Work out the finished part from the listing and answer in its coordinate system (mm). Coordinates: 2 decimals unless noted, no trailing zeros. Loops run counter-clockwise (first coordinate to the right, second up) from the corner with the lowest first, then second, coordinate; pieces in that order, holes last.
```python
from build123d import *

# Parameters (mm, degrees)
F0_W     = 75
F0_H     = 40
F1_DEPTH = 3
F3_D     = 5.5
F4_D     = 3.3


with BuildPart() as f1:
    # F0 (on Front) → F1 (new body)
    with BuildSketch(Plane.XZ):
        with Locations((37.5, 20)):
            Rectangle(F0_W, F0_H)
    extrude(amount=-F1_DEPTH)

    # F3 (through all)
    with Locations(Plane.XZ):
        with Locations((12.5, 5), (62.5, 5)):
            Hole(F3_D / 2)

    # F4 (through all)
    with Locations(Plane.XZ):
        with Locations((11.75, 36.590098), (31.05, 36.590098), (43.94, 36.590098), (63.24, 36.590098)):
            Hole(F4_D / 2)


solid = f1.part
```
1. Straight lines are drawn through the part: probe 1 along X at (y, z) = (1.05, 36.5); probe 2 along Z at (x, y) = (62, 2.35); probe 3 along Z at (x, y) = (12.5, 1.3). For each, find the intervals that lie inside material, in ascending order.
2. A cutting plane is placed at D-D, the plane y = 1.7. Give the vertices of the cut face in (x, z).
3. A cutting plane is placed at B-B, the plane z = 7. Give the vertices of the cut face in (x, y).
4. Each of these flat-tipped pins is pushed along its axis until it touches: P1, Ø4.5, axis at x = 43.94, z = 36.59, coming from the +Y side; P2, Ø2, axis at x = 63.24, z = 36.59, coming from the -Y side (3 decimals). Where does it stop, or does it pass through?
5. A cutting plane is placed at A-A, the plane x = 43.94. Give the vertices of the cut face in (y, z), then the cut area to 3 significant figures.
6. A cutting plane is placed at C-C, the plane x = 63.24. Give the vertices of the cut face in (y, z), then the cut area to 3 significant figures.
7. Determine the mould class of faces 1 (the flat face through (0, 1, 20)), 2 (the cylindrical face through (32.266, 1.521, 37.705)), 3 (the flat face through (37, 1, 40)) for opening direction X: released by +X, released by -X, zero draft, split by the parting line, or undercut.
Answers below:
1. probe 1: x = 0 to 10.1, 13.4 to 29.4, 32.7 to 42.29, 45.59 to 61.59, 64.89 to 75
1. probe 2: z = 0 to 2.3, 7.7 to 35.5, 37.68 to 40
1. probe 3: z = 0 to 2.25, 7.75 to 35.12, 38.06 to 40
2. outline: (0, 0) - (75, 0) - (75, 40) - (0, 40) - close; hole circle Ø5.5 at (12.5, 5); hole circle Ø3.3 at (11.75, 36.59); hole circle Ø3.3 at (31.05, 36.59); hole circle Ø3.3 at (43.94, 36.59); hole circle Ø5.5 at (62.5, 5); hole circle Ø3.3 at (63.24, 36.59)
3. outline: (0, 0) - (10.61, 0) - (10.61, 3) - (0, 3) - close; (14.39, 0) - (60.61, 0) - (60.61, 3) - (14.39, 3) - close; (64.39, 0) - (75, 0) - (75, 3) - (64.39, 3) - close
4. P1: stops at y = 3
4. P2: passes through
5. outline: (0, 0) - (3, 0) - (3, 34.94) - (0, 34.94) - close; (0, 38.24) - (3, 38.24) - (3, 40) - (0, 40) - close
5. area: 110 mm2
6. outline: (0, 0) - (3, 0) - (3, 2.35) - (0, 2.35) - close; (0, 7.65) - (3, 7.65) - (3, 34.94) - (0, 34.94) - close; (0, 38.24) - (3, 38.24) - (3, 40) - (0, 40) - close
6. area: 94.2 mm2
7. face 1: released by -X
7. face 2: undercut
7. face 3: zero draft
